Design review of the part built by this model. Coordinates are the model's own, in mm. A direction names the side the tool comes from. Coordinates: 2 decimals unless noted, no trailing zeros. Loops run counter-clockwise (first coordinate to the right, second up) from the corner with the lowest first, then second, coordinate; pieces in that order, holes last. Notation, with made-up numbers: (6, 70) -> (12, 70) arc R9 cw to (12, 78) -> close; hole circle Ø10 at (4, -19). An arc over 180 degrees is marked (long way). Use CSV: the item, a comma, the result in double quotes.
```python
from build123d import *

# Parameters (mm, degrees)
BOSS_EXTRUDE1_DEPTH      = 25.4
FILLET1_R                = 12.7
BOSS_EXTRUDE2_DEPTH      = 76.2
BOSS_EXTRUDE2_DEPTH_BACK = 31.75
SKETCH3_R                = 1.5875
FILLET2_R                = 6.35
SKETCH4_R                = 3.175
CUT_EXTRUDE2_DEPTH       = 12.7


with BuildPart() as part:
    # Sketch1 → Boss-Extrude1 (new body)
    with BuildSketch(Plane(origin=(0, 0, 0), x_dir=(1, 0, 0), z_dir=(0, 1, 0))):
        Polygon((-0.79375, 50.8), (-0.79375, 25.4), (0, 0), (0.79375, 25.4), (0.79375, 50.8), (0, 76.2), align=None)
    extrude(amount=BOSS_EXTRUDE1_DEPTH)

    # Fillet1
    # the kernel refuses this fillet: 12.7 mm, written as the material it takes off along each edge
    with BuildSketch(Plane(origin=(-0.79375, -0.495972692, -25.4), x_dir=(0, 0, -1), z_dir=(0, 1, 0)), Plane(origin=(0.79375, -0.495972692, -50.8), x_dir=(0, 0, 1), z_dir=(0, 1, 0)), Plane(origin=(0.79375, -0.495972692, -25.4), x_dir=(-0.031234752377718417, 0, 0.9995120760870789), z_dir=(0, 1, 0))) as fillet1_piece_1:
        with BuildLine():
            CenterArc((FILLET1_R * 0.0156211871642, -FILLET1_R), FILLET1_R, 90, 1.789910608)
            Line((-FILLET1_R * 0.0156135652135, -FILLET1_R * 0.000487923912921), (0, 0))
            Line((0, 0), (FILLET1_R * 0.0156211871642, 0))
        make_face()
    extrude(amount=26.391945385, mode=Mode.SUBTRACT)
    with BuildSketch(Plane(origin=(-0.79375, -0.495972692, -50.8), x_dir=(0, 0, 1), z_dir=(0, 1, 0))) as fillet1_piece_2:
        with BuildLine():
            CenterArc((FILLET1_R * 0.0156211871642, FILLET1_R), FILLET1_R, 268.210089392, 1.789910608)
            Line((-FILLET1_R * 0.0156135652135, FILLET1_R * 0.000487923912921), (0, 0))
            Line((0, 0), (FILLET1_R * 0.0156211871642, 0))
        make_face()
    extrude(amount=26.391945385, mode=Mode.SUBTRACT)

    # Sketch3 → Boss-Extrude2 (add, two sides: drawn at the far end of the back side and taken through both)
    with BuildSketch(Plane.XY.offset(-BOSS_EXTRUDE2_DEPTH_BACK)):
        with Locations((0, 1.5875)):
            Circle(SKETCH3_R)
    extrude(amount=BOSS_EXTRUDE2_DEPTH + BOSS_EXTRUDE2_DEPTH_BACK)

    # Fillet2
    # the kernel refuses this fillet: 6.35 mm, written as the material it adds along each edge
    with BuildSketch(Plane(origin=(-0.79375, 18.837315329, -31.75), x_dir=(0, 0, -1), z_dir=(0, -1, 0))) as fillet2_piece_1_section:
        with BuildLine():
            CenterArc((FILLET2_R, -FILLET2_R), FILLET2_R, 90, 90)
            Line((0, -FILLET2_R), (0, 0))
            Line((0, 0), (FILLET2_R, 0))
        make_face()
    fillet2_piece_1 = extrude(amount=34.499630657, mode=Mode.PRIVATE)
    fillet2_piece_1 = fillet2_piece_1 & Plane(origin=(0, 1.5875, -34.046856279), x_dir=(1, 0, 0), z_dir=(0, 0, 1)) * Cylinder(1.5875, 95, mode=Mode.PRIVATE)
    add(fillet2_piece_1)
    with BuildSketch(Plane(origin=(0.79375, -15.662315329, -31.75), x_dir=(0, 0, -1), z_dir=(0, 1, 0))) as fillet2_piece_2_section:
        with BuildLine():
            CenterArc((FILLET2_R, -FILLET2_R), FILLET2_R, 90, 90)
            Line((0, -FILLET2_R), (0, 0))
            Line((0, 0), (FILLET2_R, 0))
        make_face()
    fillet2_piece_2 = extrude(amount=34.499630657, mode=Mode.PRIVATE)
    fillet2_piece_2 = fillet2_piece_2 & Plane(origin=(0, 1.5875, -34.046857324), x_dir=(1, 0, 0), z_dir=(0, 0, 1)) * Cylinder(1.5875, 95, mode=Mode.PRIVATE)
    add(fillet2_piece_2)

    # Sketch4 → Cut-Extrude2 (cut)
    with BuildSketch(Plane(origin=(0, 0, 0), x_dir=(1, 0, 0), z_dir=(0, 1, 0))):
        with Locations((0, 6.35)):
            Circle(SKETCH4_R)
    extrude(amount=CUT_EXTRUDE2_DEPTH, mode=Mode.SUBTRACT)


solid = part.part
```
Item 1: Add section A-A (y = 7.5). Give the boundary of the cut face in (x, z) (3 decimals).
Checked values:
outline,"(-0.794, -50.602) arc R12.7 ccw to (-0.788, -50.998) -> (0, -76.2) -> (0.788, -50.998) arc R12.7 ccw to (0.794, -50.602) -> (0.794, -25.598) arc R12.7 ccw to (0.788, -25.202) -> (0.297, -9.511) arc R3.175 cw to (-0.297, -9.511) -> (-0.788, -25.202) arc R12.7 ccw to (-0.794, -25.598) -> close; (-0.099, -3.177) arc R3.175 cw to (0.099, -3.177) -> (0, 0) -> close"
Item 2: To check wall thickness, follow line 1 along X through (y, z) = (8.25, -42); line 2 along Y through (x, z) = (-0.35, 30); line 3 along Y through (x, z) = (0.2, 57). State the ranges of each line that lie inside material, in increasing order.
Checked values:
line 1,"-0.79 to 0.79"
line 2,"0.04 to 3.14"
line 3,"0.01 to 3.16"
Item 3: Machinability: for faces 5 (the face through (0, 2, 76.2)), 6 (the face through (-0.21, 3.16, 35.74)), which of the approach directions +Z, -Z, +X, -X, +Y, -Y give a long, thin tool a straight path to every point of the face, cutting with its end or side? Answer none if there is none.
Checked values:
face 5,"+Z, +X, -X, +Y, -Y"
face 6,"+Z"
Item 4: Draft analysis for pull direction X (two halves, no side actions). For faces 1 (the face through (0.008, 4.439, -9.525)), 2 (the face through (0.912, 1.568, -36.882)), 3 (the face through (-0.008, 2.557, -3.175)), 4 (the face through (-0.912, 1.607, -36.882)), state which applies: pulls with the +X half, pulls with the -X half, needs draft (parallel to the pull), parting line crosses it, or undercut.
Checked values:
face 1,"undercut"
face 2,"pulls with the +X half"
face 3,"undercut"
face 4,"pulls with the -X half"
Item 5: Add section C-C (z = 57.5). Give the boundary of the cut face in (x, y) (1 decimal).
Checked values:
outline,"circle Ø3.2 at (0, 1.6)"
Item 6: Add section B-B (y = 18.5). Give the boundary of the cut face in (x, z), then the cut area to 3 significant figures.
Checked values:
outline,"(-0.79, -51) -> (0, -76.2) -> (0.79, -51) arc R12.7 ccw to (0.79, -50.6) -> (0.79, -25.6) arc R12.7 ccw to (0.79, -25.2) -> (0, 0) -> (-0.79, -25.2) arc R12.7 ccw to (-0.79, -25.6) -> (-0.79, -50.6) arc R12.7 ccw to start"
area,"80.6 mm^2"
Item 7: Clearance check with flat-ended pins moving along their axes: pin 1 (6 mm diameter, centred on y = 12.5, z = -42, fed in from +X); pin 2 (5 mm diameter, centred on y = 15, z = -36.5, fed in from -X); pin 3 (0.5 mm diameter, centred on x = 0, z = -7.5, fed in from -Y). State where each tip first meets the part, or that it passes through.
Checked values:
pin 1,"x = 0.79"
pin 2,"x = -0.79"
pin 3,"y = 12.7"
